Autodesk Inventor part; units mm, degrees
ref_plane "YZ Plane" through (0, 0, 0) normal (1, 0, 0) x (0, 1, 0)
ref_plane "XZ Plane" through (0, 0, 0) normal (0, 1, 0) x (-1, 0, 0)
ref_plane "XY Plane" through (0, 0, 0) normal (0, 0, 1) x (1, 0, 0)
sketch "Esquisse1" plane through (0, 0, 0) normal (0, 0, 1) x (1, 0, 0)
  line L0 (0, 0) -> (17.5, 0)
  line L1 (17.5, 0) -> (17.5, 35)
  line L2 (17.5, 35) -> (0, 35)
  line L3 (0, 35) -> (0, 0)
  dimension "d0" = 35
  dimension "d1" = 17.5
extrude "Extrusion1" add sketch "Esquisse1" along normal blind 2
sketch "Esquisse2" plane through (0, 0, 2) normal (0, 0, 1) x (1, 0, 0)
  line L0 (0, 0) -> (17.5, 0)
  line L1 (17.5, 35) -> (0, 35)
  line L2 (0, 35) -> (0, 0)
  line L3 (0, 29.6) -> (11.43, 29.6)
  line L4 (11.43, 29.6) -> (11.43, 5.4)
  line L5 (11.43, 5.4) -> (0, 5.4)
  line L6 (0, 5.4) -> (0, 29.6)
  line L7 (11.43, 29.6) -> (11.43, 35) construction
  line L8 (11.43, 5.4) -> (11.43, 0) construction
  circle A0 centre (2.794, 31.25) radius 1.3
  circle A1 centre (8.636, 31.25) radius 1.3
  line L9 (11.43, 17.5) -> (0, 17.5) construction
  circle A2 centre (2.8364, 3.75) radius 1.3
  circle A3 centre (8.5936, 3.75) radius 1.3
  line L10 (8.5936, 3.75) -> (2.8364, 3.75) construction
  line L11 (8.636, 31.25) -> (2.794, 31.25) construction
  line L12 (5.715, 31.25) -> (5.715, 17.5) construction
  line L13 (5.715, 17.5) -> (5.715, 3.75) construction
  line L14 (2.794, 31.25) -> (0, 31.25) construction
  line L15 (8.636, 31.25) -> (11.43, 31.25) construction
  dimension "d4" = 24.2
  dimension "d6" = 11.43
  dimension "d7" = 5.842
  dimension "d8" = 27.5
  dimension "d9" = 2.6
extrude "Extrusion2" cut sketch "Esquisse2" against normal blind 4.5
sketch "Esquisse3" plane through (0, 0, 2) normal (0, 0, 1) x (1, 0, 0)
  line L0 (0, 0) -> (17.5, 0)
  line L1 (17.5, 35) -> (13, 35)
  line L2 (13, 35) -> (13, 0)
  line L3 (13, 0) -> (17.5, 0)
  line L4 (17.5, 0) -> (17.5, 35)
  dimension "d12" = 4.5
extrude "Extrusion3" add sketch "Esquisse3" along normal blind 10
sketch "Esquisse6" plane through (0, 0, 12) normal (0, 0, 1) x (1, 0, 0)
  line L0 (13, 0) -> (17.5, 0) construction
  line L1 (17.5, 0) -> (17.5, 35) construction
  line L2 (17.5, 35) -> (13, 35) construction
  line L3 (13, 35) -> (13, 0) construction
  line L4 (13, 26.5) -> (17.5, 26.5)
  line L5 (17.5, 26.5) -> (17.5, 8.5)
  line L6 (17.5, 8.5) -> (13, 8.5)
  line L7 (13, 8.5) -> (13, 26.5)
  line L8 (15.25, 26.5) -> (15.25, 35) construction
  line L9 (15.25, 8.5) -> (15.25, 0) construction
  point P0 (0, 0)
  dimension "d28" = 18
extrude "Extrusion6" add sketch "Esquisse6" along normal blind 8
fillet "Congé2" radius 5 2 edges at (15.25, 0, 12) (15.25, 35, 12)
fillet "Congé3" radius 5 4 edges at (15.25, 26.5, 12) (15.25, 8.5, 12) (15.25, 26.5, 20) (15.25, 8.5, 20)
sketch "Esquisse4" plane through (17.5, 0, 0) normal (1, 0, 0) x (0, 0, -1)
  line L0 (0, 0) -> (0, 35) construction
  line L1 (0, 35) -> (-12, 35) construction
  line L2 (0, 0) -> (-12, 0) construction
  line L3 (-27.5, 30.05) -> (-12.5, 30.05)
  line L4 (-12.5, 30.05) -> (-12.5, 20.05)
  line L5 (-12.5, 20.05) -> (-2.5, 20.05)
  line L6 (-2.5, 20.05) -> (-2.5, 14.95)
  line L7 (-2.5, 14.95) -> (-12.5, 14.95)
  line L8 (-12.5, 14.95) -> (-12.5, 4.95)
  line L9 (-12.5, 4.95) -> (-27.5, 4.95)
  line L10 (-27.5, 4.95) -> (-27.5, 30.05)
  line L11 (-7.5, 20.05) -> (-7.5, 35) construction
  line L12 (-7.5, 14.95) -> (-7.5, 0) construction
  dimension "d15" = 10
  dimension "d17" = 5.1
  dimension "d18" = 2.5
  dimension "d19" = 15
extrude "Extrusion4" cut sketch "Esquisse4" against normal blind 2.5
sketch "Esquisse5" plane through (15, 0, 0) normal (1, 0, 0) x (0, 0, -1)
  line L0 (-12.5, 29.1009) -> (-12.5, 20.05) construction
  circle A0 centre (-15.5, 17.5) radius 1.5
  line L1 (-15.5, 17.5) -> (-12.5, 20.05) construction
  line L2 (-15.5, 17.5) -> (-12.5, 14.95) construction
  point P0 (-12.5, 4.95)
  point P1 (-12.5, 30.05)
  point P2 (0, 0)
  point P3 (-12.5, 29)
  dimension "d22" = 3
  dimension "d23" = 3
extrude "Extrusion5" cut sketch "Esquisse5" against normal up to next
fillet "Congé1" radius 2 1 edges at (17.5, 17.5, 0)
fillet "Congé4" radius 1 1 edges at (13, 17.5, 2)
properties part number "Pantilt"
Build history of the part. All positions in model axes, mm. A direction names the side the tool comes from. Round coordinates to 2 decimals unless told otherwise and drop trailing zeros. Write each loop counter-clockwise with the first axis right and the second up, starting at its lowest first coordinate (ties: lowest second). Pieces come first, ordered by that corner, then holes. Notation, with made-up numbers: (13, -28.5) - (50, -28.5) arc R18 ccw to (50, -21.5) - close; hole circle Ø5 at (-8.75, 48). An arc over 180 degrees is marked (long way). Answer as CSV lines item,"result".
Q1. Cut at B-B (y = 17.5). Write the cut outline in (x, z), and give its area (3 significant figures).
Report:
outline,"(11.43, 0) - (15.5, 0) arc R2 ccw to (17.5, 2) - (17.5, 2.5) - (15, 2.5) - (15, 14) - (13, 14) - (13, 3) arc R1 cw to (12, 2) - (11.43, 2) - close; (13, 17) - (15, 17) - (15, 20) - (13, 20) - close"
area,"42.7 mm^2"
Q2. Cut at D-D (y = 3.75). Write the cut outline in (x, z).
Report:
outline,"(0, 0) - (1.54, 0) - (1.54, 2) - (0, 2) - close; (4.14, 0) - (7.29, 0) - (7.29, 2) - (4.14, 2) - close; (9.89, 0) - (15.5, 0) arc R2 ccw to (17.5, 2) - (17.5, 11.84) - (13, 11.84) - (13, 3) arc R1 cw to (12, 2) - (9.89, 2) - close"
Q3. Cut at A-A (x = 5). Write the cut outline in (y, z), and give its area (3 significant figures).
Report:
outline,"(0, 0) - (5.4, 0) - (5.4, 2) - (0, 2) - close; (29.6, 0) - (35, 0) - (35, 2) - (29.6, 2) - close"
area,"21.6 mm^2"
Q4. Tool access for faces 1 (the flat face through (13, 18, 9)), 2 (the flat face through (11, 35, 1)), 3 (the flat face through (6, 29.6, 1)), 4 (the flat face through (14, 18, 20)), 5 (the flat face through (16, 18, 2.5)): list every direction of +Z, -Z, +X, -X, +Y, -Y with a clear straight run to the whole face (end or side of a thin tool).
Report:
face 1,"+Z, -X, +Y, -Y"
face 2,"+Z, -Z, +X, -X, +Y"
face 3,"+Z, -Z, -X"
face 4,"+Z, +X, -X, +Y, -Y"
face 5,"+Z, +X"
Q5. Cut at C-C (z = 5). Write the cut outline in (x, y), and give its area (3 significant figures).
Report:
outline,"(13, 0) - (17.5, 0) - (17.5, 14.95) - (15, 14.95) - (15, 20.05) - (17.5, 20.05) - (17.5, 35) - (13, 35) - close"
area,"145 mm^2"
Q6. Drop flat-ended pins along their axis: pin 1 (1.6 mm diameter, centred on y = 20.5, z = 0.5, fed in from -X); pin 2 (3 mm diameter, centred on x = 8.636, y = 31.25, fed in from +Z); pin 3 (8 mm diameter, centred on x = 14.5, z = 17, fed in from -Y). Give the stop position or say it passes through.
Report:
pin 1,"stops at x = 11.43"
pin 2,"stops at z = 2"
pin 3,"stops at y = 6.65"
Q7. Drill centre lines: probe 1 along Z at (x, y) = (12, 13); probe 2 along X at (y, z) = (11.5, 4.5); probe 3 along Y at (x, z) = (15.25, 11.5). Where is each one in solid material? Low to high. Write a range as [from, to].
Report:
probe 1,"z = [0, 2]"
probe 2,"x = [13, 17.5]"
probe 3,"y = [2.82, 14.95], [20.05, 32.18]"
Q8. Pull direction X, two halves, no side cores. Call faces 6 (the flat face through (11.43, 18, 1)), 7 (the flat face through (16, 25, 12.5)), 8 (the cylindrical face through (7.56, 2.96, 1.01)): +X half, -X half, draft (parallel to the pull), parting line (faces both ways), or undercut.
Report:
face 6,"-X half"
face 7,"draft"
face 8,"undercut"
